Check sheet for the modelled part. Datum: model origin and axes. Units: mm. Face numbers are marked on the shaded views. A direction names the side the tool comes from. Round coordinates to 2 decimals unless told otherwise and drop trailing zeros. Write each loop counter-clockwise with the first axis right and the second up, starting at its lowest first coordinate (ties: lowest second). Pieces come first, ordered by that corner, then holes. Notation, with made-up numbers: (21.5, 57) -> (79.5, 57) arc R26 cw to (79.5, 96) -> close; hole circle Ø4 at (41.5, 73.25). An arc over 180 degrees is marked (long way). One line per item, written item: value. Start each with the question number.
```python
from build123d import *

# Parameters (mm, degrees)
CBODY_DEPTH            = 7
CBODY_DEPTH_BACK       = 5.6
CBODY_SKETCH_R         = 6.7
CBODY_CHAMFER_SIZE     = 0.25
THREAD_OFFSET_SKETCH_R = 6.5
THREAD_OFFSET_DEPTH    = 1
HEAD_SKETCH_R          = 5
HEAD_DEPTH             = 5.1
HEX_2_DEPTH            = 3
TUBE_START             = -13.3
TUBE_SKETCH_R          = 3.175
TUBE_DEPTH             = 13.3
TUBE_FILLET_R          = 0.5
PROFILE_PORT_R         = 1.5875


with BuildPart() as part:
    # CBody_Sketch → CBody (new, two sides: drawn at the far end of the back side and taken through both)
    with BuildSketch(Plane(origin=(0, 0, 0), x_dir=(1, 0, 0), z_dir=(0, 1, 0)).offset(-CBODY_DEPTH_BACK)):
        with Locations(Location((0, 0, 0), (0, 0, 270))):
            Circle(CBODY_SKETCH_R)
    extrude(amount=CBODY_DEPTH + CBODY_DEPTH_BACK)

    # CBody_Chamfer
    cbody_chamfer_edges = [part.edges().sort_by_distance(p)[0] for p in [
        (0, 7, -6.7),
    ]]
    chamfer(cbody_chamfer_edges, length=CBODY_CHAMFER_SIZE)

    # Thread_Offset_Sketch → Thread_Offset (add)
    with BuildSketch(Plane(origin=(0, -5.6, 0), x_dir=(-1, 0, 0), z_dir=(0, 1, 0))):
        with Locations(Location((0, 0, 0), (0, 0, 90))):
            Circle(THREAD_OFFSET_SKETCH_R)
    extrude(amount=-THREAD_OFFSET_DEPTH)

    # Thread_Sketch → Thread (revolve)
    with BuildSketch(Plane.XY, mode=Mode.PRIVATE) as thread_sk:
        Polygon((-5.24727057, -6.6), (-5.026624869, -13.7), (0, -13.7), (0, -6.6), align=None)
    revolve(thread_sk.sketch.rotate(Axis((0, 0, 0), (0, -1, 0)), 270), axis=Axis((0, 0, 0), (0, -1, 0)))

    # Thread_Chamfer: read off the stored shape, not the designer's step
    # Thread_Chamfer outline → Thread_Chamfer (revolve, cut)
    with BuildSketch(Plane.XY):
        Polygon((5.03464327, -13.441981598), (4.776624869, -13.7), (5.03464327, -13.7), align=None)
    revolve(axis=Axis((0, 0, 0), (0, 1, 0)), mode=Mode.SUBTRACT)

    # Head_Sketch → Head (add)
    with BuildSketch(Plane(origin=(0, 7, 0), x_dir=(-1, 0, 0), z_dir=(0, 1, 0))):
        with Locations(Location((0, 0, 0), (0, 0, 90))):
            Circle(HEAD_SKETCH_R)
    extrude(amount=HEAD_DEPTH)

    # Hex_Sketch → Hex 2 (cut)
    with BuildSketch(Plane(origin=(0, 12.1, 0), x_dir=(-1, 0, 0), z_dir=(0, 1, 0))):
        Polygon((-1.833087105, 3.175), (-3.666174209, 0), (-1.833087105, -3.175), (1.833087105, -3.175), (3.666174209, 0), (1.833087105, 3.175), align=None)
    extrude(amount=-HEX_2_DEPTH, mode=Mode.SUBTRACT)

    # RBody_Sketch → RBody (revolve)
    with BuildSketch(Plane(origin=(0, 0, 0), x_dir=(1, 0, 0), z_dir=(0, 1, 0))):
        Polygon((0, 0), (2.915618859, -5.05), (8.9, -5.05), (9.188675135, -5.55), (18.2, -5.55), (18.2, 0), align=None)
    revolve(axis=Axis((-16.33553342, 0, 0), (1, 0, 0)))

    # Release_Sketch → Release (revolve)
    with BuildSketch(Plane(origin=(0, 0, 0), x_dir=(1, 0, 0), z_dir=(0, 1, 0)), mode=Mode.PRIVATE) as release_sk:
        with BuildLine():
            Line((18.2, 0), (18.2, 3.925))
            Line((18.2, 3.925), (19.1, 3.925))
            Line((19.1, 3.925), (19.1, 5.025))
            Line((19.1, 5.025), (20.1, 5.025))
            ThreePointArc((20.1, 5.025), (20.453553391, 4.878553391), (20.6, 4.525))
            Line((20.6, 4.525), (20.6, 0))
            Line((20.6, 0), (18.2, 0))
        make_face()
    revolve(release_sk.sketch.rotate(Axis((0, 0, 0), (1, 0, 0)), 180), axis=Axis((0, 0, 0), (1, 0, 0)))

    # Tube_Sketch → Tube (cut)
    with BuildSketch(Plane(origin=(20.6, 0, 0), x_dir=(0, 0, -1), z_dir=(1, 0, 0)).offset(TUBE_START)):
        Circle(TUBE_SKETCH_R)
    extrude(amount=TUBE_DEPTH, mode=Mode.SUBTRACT)

    # Tube_Fillet
    tube_fillet_edges = [part.edges().sort_by_distance(p)[0] for p in [
        (20.6, 0, 3.175),
    ]]
    fillet(tube_fillet_edges, radius=TUBE_FILLET_R)

    # Port: sweep along a path in Path Port
    with BuildLine(Plane.XY) as port_path:
        Line((20.6, 0), (2, 0))
        ThreePointArc((2, 0), (0.585786438, -0.585786438), (0, -2))
        Line((0, -2), (0, -13.7))
    # Profile Port → Port (sweep, cut)
    with BuildSketch(Plane(origin=(20.6, 0, 0), x_dir=(0, 0, -1), z_dir=(1, 0, 0))):
        Circle(PROFILE_PORT_R)
    sweep(path=port_path.line, mode=Mode.SUBTRACT)


solid = part.part
```
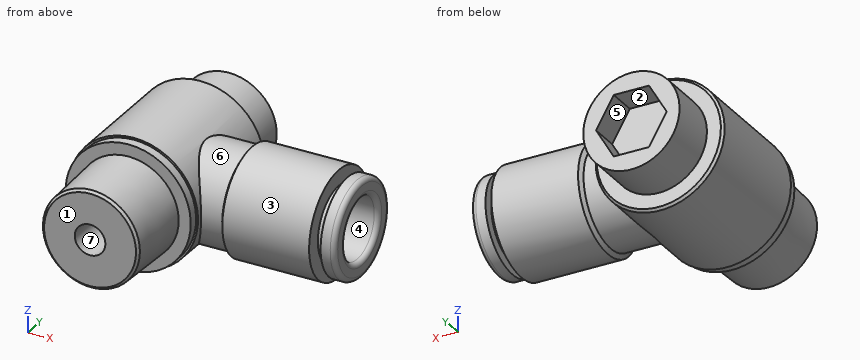
1. Depth check by flat-ended pin: pin 1 Ø1.9 at (y, z) = (1.5, 0.5) entering from +X; pin 2 Ø3.5 at (x, y) = (1, 11) entering from -Z; pin 3 Ø5 at (x, z) = (0, 0) entering from +Y. Enter the tip coordinate at first touch or a pass-through.
2. Material ranges on probe 1 along X at (y, z) = (-4.5, 0); probe 2 along X at (y, z) = (-5.25, 0); probe 3 along Z at (x, y) = (4.95, 0), recorded low to high.
3. Cross-section at B-B (y = -7). Record the cut outline in (x, z) (1 decimal).
4. Access from +Z, -Z, +X, -X, +Y, -Y to the whole of each face (thin tool, end or side, straight path). Record for the marked faces 4, 5, 6 and 7.
5. Cross-section at A-A (x = 14.25). Record the cut outline in (y, z) (3 decimals), plus the area to 3 significant figures.
6. Release check for a two-part mould opening along Z. For the marked faces 1, 2 and 3 record: +Z half, -Z half, draft (parallel to the pull), parting line (faces both ways), or undercut.
Working result:
1. pin 1: stops at x = 7.3
1. pin 2: stops at z = -5
1. pin 3: stops at y = 9.1
2. probe 1: x = -6.7 to -1.59, 1.59 to 18.2, 19.1 to 20.6
2. probe 2: x = -6.7 to -1.59, 1.59 to 6.7, 9.02 to 18.2
2. probe 3: z = -5.05 to -1.59, 1.59 to 5.05
3. outline: circle Ø10.5 at (0, 0); hole circle Ø3.2 at (0, 0)
4. face 4: +X
4. face 5: +Y
4. face 6: none
4. face 7: -Y
5. outline: circle Ø11.1 at (0, 0); hole circle Ø6.35 at (0, 0)
5. area: 65.1 mm^2
6. face 1: draft
6. face 2: undercut
6. face 3: parting line
